```python
from build123d import *

# Parameters (mm, degrees)
ESTRUSIONE_ESTRUSIONE1_DEPTH      = 48
ESTRUSIONE_ESTRUSIONE1_DEPTH_BACK = 6
SCHIZZO2_W                        = 2
SCHIZZO2_H                        = 45
ESTRUSIONE_ESTRUSIONE2_DEPTH      = 5
CORPO_SPOSTA_COPIA1_START         = 18.633322101
CORPO_SPOSTA_COPIA1_OUTLINE_W     = 2
CORPO_SPOSTA_COPIA1_OUTLINE_H     = 42
CORPO_SPOSTA_COPIA1_DEPTH         = 34.028742836
CORPO_SPOSTA_COPIA1_2_OUTLINE_W   = 2
CORPO_SPOSTA_COPIA1_2_OUTLINE_H   = 6
CORPO_SPOSTA_COPIA1_2_DEPTH       = 5
CORPO_SPOSTA_COPIA1_START_2       = 47.662064937
CORPO_SPOSTA_COPIA1_3_OUTLINE_W   = 2
CORPO_SPOSTA_COPIA1_3_OUTLINE_H   = 6
CORPO_SPOSTA_COPIA1_3_DEPTH       = 5
CORPO_SPOSTA_COPIA1_4_OUTLINE_W   = 2
CORPO_SPOSTA_COPIA1_4_OUTLINE_H   = 45
CORPO_SPOSTA_COPIA1_4_DEPTH       = 34.028742836
CORPO_SPOSTA_COPIA1_START_3       = 23.633322101
CORPO_SPOSTA_COPIA1_5_OUTLINE_W   = 2
CORPO_SPOSTA_COPIA1_5_OUTLINE_H   = 3
CORPO_SPOSTA_COPIA1_5_DEPTH       = 24.028742836


# Read off the part's stored shape, not the designer's step: Corpo-Sposta/copia1
with BuildPart() as part:
    # Schizzo1 → Estrusione-Estrusione1 (new, two sides: drawn at the far end of the back side and taken through both)
    with BuildSketch(Plane.XY.offset(-ESTRUSIONE_ESTRUSIONE1_DEPTH_BACK)):
        Polygon((235.52839554, -38.086696659), (227.03131331, -60.562907992), (228.902090444, -61.27015117), (237.399172674, -38.793939838), align=None)
    extrude(amount=ESTRUSIONE_ESTRUSIONE1_DEPTH + ESTRUSIONE_ESTRUSIONE1_DEPTH_BACK)

    # Schizzo2 → Estrusione-Estrusione2 (add)
    with BuildSketch(Plane(origin=(16.854335152, 44.58255063, 0), x_dir=(0.9353885671687735, -0.3536215892871206, 0), z_dir=(0.3536215892871206, 0.9353885671687735, 0))):
        with Locations((234.778846635, -22.5)):
            Rectangle(SCHIZZO2_W, SCHIZZO2_H)
    estrusione_estrusione2 = extrude(amount=ESTRUSIONE_ESTRUSIONE2_DEPTH)

    # Specchia1: Estrusione-Estrusione2 across plane
    add(estrusione_estrusione2.mirror(Plane(origin=(12.605794037, 33.344444963, 0), x_dir=(0, 0, 1), z_dir=(0.35362158928712106, 0.9353885671687733, 0))))

    # Corpo-Sposta/copia1 outline → Corpo-Sposta/copia1 (cut)
    with BuildSketch(Plane(origin=(0, 0, 0), x_dir=(0.9353885671687733, -0.3536215892871211, 0), z_dir=(0.35362158928712106, 0.9353885671687733, 0)).offset(CORPO_SPOSTA_COPIA1_START)):
        with Locations((234.778846635, -27)):
            Rectangle(CORPO_SPOSTA_COPIA1_OUTLINE_W, CORPO_SPOSTA_COPIA1_OUTLINE_H)
    extrude(amount=CORPO_SPOSTA_COPIA1_DEPTH, mode=Mode.SUBTRACT)

    # Corpo-Sposta_copia1 2 outline → Corpo-Sposta_copia1 2 (cut)
    with BuildSketch(Plane(origin=(0, 0, 0), x_dir=(0.9353885671687733, -0.3536215892871211, 0), z_dir=(0.35362158928712106, 0.9353885671687733, 0)).offset(CORPO_SPOSTA_COPIA1_START)):
        with Locations((234.778846635, -3)):
            Rectangle(CORPO_SPOSTA_COPIA1_2_OUTLINE_W, CORPO_SPOSTA_COPIA1_2_OUTLINE_H)
    extrude(amount=CORPO_SPOSTA_COPIA1_2_DEPTH, mode=Mode.SUBTRACT)

    # Corpo-Sposta_copia1 3 outline → Corpo-Sposta_copia1 3 (cut)
    with BuildSketch(Plane(origin=(0, 0, 0), x_dir=(0.9353885671687733, -0.3536215892871211, 0), z_dir=(0.35362158928712106, 0.9353885671687733, 0)).offset(CORPO_SPOSTA_COPIA1_START_2)):
        with Locations((234.778846635, -3)):
            Rectangle(CORPO_SPOSTA_COPIA1_3_OUTLINE_W, CORPO_SPOSTA_COPIA1_3_OUTLINE_H)
    extrude(amount=CORPO_SPOSTA_COPIA1_3_DEPTH, mode=Mode.SUBTRACT)

    # Corpo-Sposta_copia1 4 outline → Corpo-Sposta_copia1 4 (add)
    with BuildSketch(Plane(origin=(0, 0, 0), x_dir=(0.9353885671687733, -0.3536215892871211, 0), z_dir=(0.35362158928712106, 0.9353885671687733, 0)).offset(CORPO_SPOSTA_COPIA1_START)):
        with Locations((234.778846635, 22.5)):
            Rectangle(CORPO_SPOSTA_COPIA1_4_OUTLINE_W, CORPO_SPOSTA_COPIA1_4_OUTLINE_H)
    extrude(amount=CORPO_SPOSTA_COPIA1_4_DEPTH)

    # Corpo-Sposta_copia1 5 outline → Corpo-Sposta_copia1 5 (add)
    with BuildSketch(Plane(origin=(0, 0, 0), x_dir=(0.9353885671687733, -0.3536215892871211, 0), z_dir=(0.35362158928712106, 0.9353885671687733, 0)).offset(CORPO_SPOSTA_COPIA1_START_3)):
        with Locations((234.778846635, 46.5)):
            Rectangle(CORPO_SPOSTA_COPIA1_5_OUTLINE_W, CORPO_SPOSTA_COPIA1_5_OUTLINE_H)
    extrude(amount=CORPO_SPOSTA_COPIA1_5_DEPTH)


solid = part.part
```
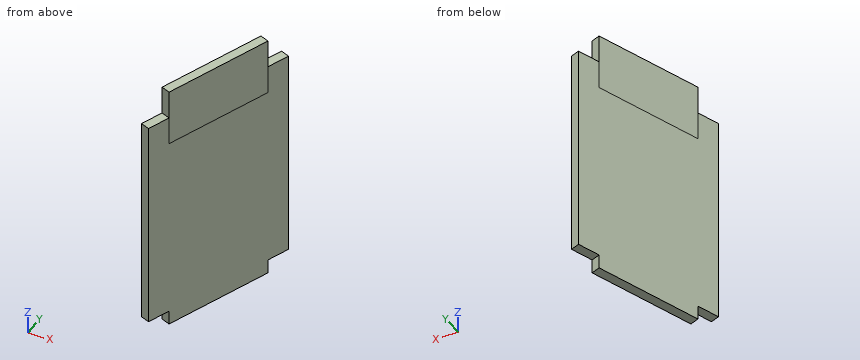
Verification items for the finished model (mm, model axes). Coordinates: 2 decimals unless noted, no trailing zeros. Write each loop counter-clockwise with the first axis right and the second up, starting at its lowest first coordinate (ties: lowest second). Pieces come first, ordered by that corner, then holes. Notation, with made-up numbers: (-13.5, 8) - (-7.5, 8) arc R19 ccw to (-7.5, 44) - close; hole circle Ø8 at (70, 13). An arc over 180 degrees is marked (long way). Write item = value, one per line.
Q1. Cross-section at A-A (z = -39.5). Enter the section's corners in (x, y).
Answer:
outline = (225.26, -65.24) - (227.13, -65.95) - (239.17, -34.12) - (237.3, -33.41) - close
Q2. Cross-section at D-D (y = -62.5). Enter the section's corners in (x, z), plus the area to 3 significant figures.
Answer:
outline = (226.3, -45) - (228.44, -45) - (228.44, 0) - (226.3, 0) - close
area = 96.2 mm²
Q3. Material ranges on L1, parallel to Z at x = 236.25, y = -37.5; L2, parallel to X at y = -61.5, z = -19; L3, parallel to X at y = -63, z = -31, recorded low to high. Write a range as from..to.
Answer:
L1 = -45..0
L2 = 226.68..228.82
L3 = 226.11..228.25
Q4. Go/stop test with flat-tipped pins: pin 1 Ø3 at (x, y) = (237.5, -36.5) entering from +Z; pin 2 Ø8 at (y, z) = (-46.5, 0) entering from +X; pin 3 Ø8 at (y, z) = (-40.5, -33.5) entering from +X. Record where each tip stops, or that it passes through.
Answer:
pin_1 = 0
pin_2 = 236
pin_3 = 238.27
Q5. Cross-section at C-C (x = 227.75). Enter the section's corners in (y, z).
Answer:
outline = (-64.32, -45) - (-60.83, -45) - (-60.83, -48) - (-58.66, -48) - (-58.66, 6) - (-60.83, 6) - (-60.83, 0) - (-64.32, 0) - close
Q6. Cross-section at B-B (y = -45.5). Enter the section's corners in (x, z), plus the area to 3 significant figures.
Answer:
outline = (232.73, -48) - (234.86, -48) - (234.86, 6) - (232.73, 6) - close
area = 115 mm²
